Check sheet for the modelled part. Datum: model origin and axes. Units: mm. A direction names the side the tool comes from. Coordinates: 2 decimals unless noted, no trailing zeros. Loops run counter-clockwise (first coordinate to the right, second up) from the corner with the lowest first, then second, coordinate; pieces in that order, holes last.
```python
from build123d import *

# Parameters (mm, degrees)
SALIENTE_EXTRUIR1_DEPTH    = 12
CORTAR_EXTRUIR1_DEPTH      = 6
CROQUIS5_R                 = 1.875
CORTAR_EXTRUIR2_DEPTH      = 7
CORTAR_EXTRUIR2_DEPTH_BACK = 7
CROQUIS6_W                 = 80
CROQUIS6_H                 = 8
CROQUIS6_R                 = 1.875
SALIENTE_EXTRUIR4_DEPTH    = 3
CORTAR_EXTRUIR3_DEPTH      = 8


with BuildPart() as part:
    # Croquis1 → Saliente-Extruir1 (new body)
    with BuildSketch(Plane(origin=(0, 0, 0), x_dir=(1, 0, 0), z_dir=(0, 1, 0))):
        with BuildLine():
            Line((-40, 11), (40, 11))
            ThreePointArc((40, 11), (51, 0), (40, -11))
            Line((40, -11), (-40, -11))
            ThreePointArc((-40, -11), (-51, 0), (-40, 11))
        make_face()
        with BuildLine():
            Line((-40, 3), (40, 3))
            ThreePointArc((40, 3), (43, 0), (40, -3))
            Line((40, -3), (-40, -3))
            ThreePointArc((-40, -3), (-43, 0), (-40, 3))
        make_face(mode=Mode.SUBTRACT)
    extrude(amount=SALIENTE_EXTRUIR1_DEPTH)

    # Croquis2 → Cortar-Extruir1 (cut)
    with BuildSketch(Plane(origin=(0, 0, 0), x_dir=(1, 0, 0), z_dir=(0, 1, 0))):
        Polygon((45.4, -2.771281292), (43.8, 0), (45.4, 2.771281292), (48.6, 2.771281292), (50.2, 0), (48.6, -2.771281292), align=None)
        Polygon((-45.4, 2.771281292), (-48.6, 2.771281292), (-50.2, 0), (-48.6, -2.771281292), (-45.4, -2.771281292), (-43.8, 0), align=None)
    extrude(amount=CORTAR_EXTRUIR1_DEPTH, mode=Mode.SUBTRACT)

    # Croquis5 → Cortar-Extruir2 (cut, two sides)
    with BuildSketch(Plane.XZ.offset(-6)) as cortar_extruir2_sk:
        with Locations((-47, 0)):
            Circle(CROQUIS5_R)
        with Locations((47, 0)):
            Circle(CROQUIS5_R)
    extrude(amount=CORTAR_EXTRUIR2_DEPTH, mode=Mode.SUBTRACT)
    extrude(cortar_extruir2_sk.sketch, amount=-CORTAR_EXTRUIR2_DEPTH_BACK, mode=Mode.SUBTRACT)

    # Croquis6 → Saliente-Extruir4 (add)
    with BuildSketch(Plane(origin=(0, 12, 0), x_dir=(1, 0, 0), z_dir=(0, 1, 0))):
        with Locations((0, 7)):
            Rectangle(CROQUIS6_W, CROQUIS6_H)
        with Locations((0, -7)):
            Rectangle(CROQUIS6_W, CROQUIS6_H)
        with BuildLine():
            Line((-40, 3), (-40, 11))
            ThreePointArc((-40, 11), (-51, 0), (-40, -11))
            Line((-40, -11), (-40, -3))
            ThreePointArc((-40, -3), (-43, 0), (-40, 3))
        make_face()
        with Locations((-47, 0)):
            Circle(CROQUIS6_R, mode=Mode.SUBTRACT)
        with BuildLine():
            ThreePointArc((40, -11), (51, 0), (40, 11))
            Line((40, 11), (40, 3))
            ThreePointArc((40, 3), (43, 0), (40, -3))
            Line((40, -3), (40, -11))
        make_face()
        with Locations((47, 0)):
            Circle(CROQUIS6_R, mode=Mode.SUBTRACT)
    extrude(amount=SALIENTE_EXTRUIR4_DEPTH)

    # Croquis7 → Cortar-Extruir3 (cut)
    with BuildSketch(Plane(origin=(0, 15, 0), x_dir=(1, 0, 0), z_dir=(0, 1, 0))):
        with BuildLine():
            Line((-40, 9), (40, 9))
            ThreePointArc((40, 9), (49, 0), (40, -9))
            Line((40, -9), (-40, -9))
            ThreePointArc((-40, -9), (-49, 0), (-40, 9))
        make_face()
    extrude(amount=-CORTAR_EXTRUIR3_DEPTH, mode=Mode.SUBTRACT)


solid = part.part
```
1) Section check D-D on z = 4.75. Enter the section's corners in (x, y).
Answer sheet:
outline: (-49.92, 0) - (49.92, 0) - (49.92, 15) - (47.64, 15) - (47.64, 7) - (-47.64, 7) - (-47.64, 15) - (-49.92, 15) - close
2) Section check B-B on y = 10. Enter the section's corners in (x, z), plus the area to 3 significant figures.
Answer sheet:
outline: (-40, -11) - (40, -11) arc R11 ccw to (40, 11) - (-40, 11) arc R11 ccw to start; hole (-40, -9) - (40, -9) arc R9 ccw to (40, 9) - (-40, 9) arc R9 ccw to start
area: 446 mm2
3) Mould release check, pull along X, two halves, no side actions. Record for faces 5 (the flat face through (44.611, 2.958, 1.405)), 6 (the flat face through (1, 0, 5)), 7 (the cylindrical face through (51, 7, 0)): +X half, -X half, draft (parallel to the pull), parting line (faces both ways), or undercut.
Answer sheet:
face 5: undercut
face 6: draft
face 7: +X half
4) Depth check by flat-ended pin: pin 1 (1 mm diameter, centred on x = 47.5, y = 4, fed in from +Z); pin 2 (1.7 mm diameter, centred on x = 48, z = -1, fed in from -Y); pin 3 (1.5 mm diameter, centred on y = 7.5, z = -6, fed in from -X). Enter the tip coordinate at first touch or a pass-through.
Answer sheet:
pin 1: stops at z = 8.49
pin 2: stops at y = 6
pin 3: stops at x = -49.67
5) Section check A-A on x = -9.5. Enter the section's corners in (y, z).
Answer sheet:
outline: (0, -11) - (15, -11) - (15, -9) - (7, -9) - (7, -3) - (0, -3) - close; (0, 3) - (7, 3) - (7, 9) - (15, 9) - (15, 11) - (0, 11) - close
6) Set-up check for faces 1 (the flat face through (-1, 7, 11)), 2 (the cylindrical face through (43, 3, 0)), 3 (the flat face through (-49.389, 2.958, -1.405)), 4 (the flat face through (1, 11, 9)): record each of +Z, -Z, +X, -X, +Y, -Y from which the full face is reachable in a straight line by a thin tool's end or side.
Answer sheet:
face 1: +Z, +X, -X, +Y, -Y
face 2: +Y, -Y
face 3: -Y
face 4: +Y
7) Section check C-C on y = 3.5. Enter the section's corners in (x, z).
Answer sheet:
outline: (-40, -11) - (40, -11) arc R11 ccw to (40, 11) - (-40, 11) arc R11 ccw to start; hole (-50.2, 0) - (-48.6, -2.77) - (-45.4, -2.77) - (-43.8, 0) - (-45.4, 2.77) - (-48.6, 2.77) - close; hole (-40, -3) - (40, -3) arc R3 ccw to (40, 3) - (-40, 3) arc R3 ccw to start; hole (43.8, 0) - (45.4, -2.77) - (48.6, -2.77) - (50.2, 0) - (48.6, 2.77) - (45.4, 2.77) - close
8) Scan lines: line 1 (Z direction, x = -36, y = 3.75); line 2 (Z direction, x = -19.5, y = 9); line 3 (X direction, y = 6.25, z = -0.75). Record each from-to range of solid material in increasing order.
Answer sheet:
line 1: z = -11 to -3, 3 to 11
line 2: z = -11 to -9, 9 to 11
line 3: x = -50.97 to -48.72, -45.28 to -42.9, 42.9 to 45.28, 48.72 to 50.97
